Work out the finished part from the listing and answer in its coordinate system (mm). A direction names the side the tool comes from. Coordinates: 2 decimals unless noted, no trailing zeros. Write each loop counter-clockwise with the first axis right and the second up, starting at its lowest first coordinate (ties: lowest second). Pieces come first, ordered by that corner, then holes. Notation, with made-up numbers: (65.5, 52.25) - (106.5, 52.25) arc R37 ccw to (106.5, 89.25) - close; hole circle Ø1 at (-0.75, 13). An arc over 180 degrees is marked (long way). One line per item, written item: value.
```python
from build123d import *

# Parameters (mm, degrees)
F1_DEPTH = 3.41884
F2_R     = 0.762
F3_R     = 1.35255
F4_DEPTH = 3.41884


with BuildPart() as f1:
    # F0 (on Top) → F1 (new body)
    with BuildSketch(Plane.XY):
        with BuildLine():
            ThreePointArc((6.35, 0), (3.175, 3.175), (0, 0))
            Line((0, 0), (0, -169.139565))
            Line((0, -169.139565), (-3.174995, -174.638818))
            Line((-3.174995, -174.638818), (9.524995, -174.638818))
            Line((9.524995, -174.638818), (6.35, -169.139565))
            Line((6.35, -169.139565), (6.35, 0))
        make_face()
    extrude(amount=F1_DEPTH)

    # F2
    f2_edges = [f1.edges().sort_by_distance(p)[0] for p in [
        (9.524995, -174.638818, 1.70942),
        (-3.174995, -174.638818, 1.70942),
    ]]
    fillet(f2_edges, radius=F2_R)

    # F3 (on face) → F4 (cut, through all)
    with BuildSketch(Plane.XY.offset(3.41884)):
        with Locations((3.175, 0)):
            Circle(F3_R)
        with Locations((3.175, -85.731909)):
            Circle(F3_R)
        with Locations((3.175, -171.463818)):
            Circle(F3_R)
    extrude(amount=-F4_DEPTH, mode=Mode.SUBTRACT)


solid = f1.part
```
Item 1: Section B-B, the plane y = -155 is taken. Determine the outline of the cut face in (x, z), then the cut area to 3 significant figures.
Evaluation:
outline: (0, 0) - (6.35, 0) - (6.35, 3.42) - (0, 3.42) - close
area: 21.7 mm2
Item 2: Section A-A, the plane z = 1.3 is taken. Determine the outline of the cut face in (x, y) (3 decimals), then the cut area to 3 significant figures.
Evaluation:
outline: (-2.515, -173.496) arc R0.762 ccw to (-1.855, -174.639) - (8.205, -174.639) arc R0.762 ccw to (8.865, -173.496) - (6.35, -169.14) - (6.35, 0) arc R3.175 ccw to (0, 0) - (0, -169.14) - close; hole circle Ø2.705 at (3.175, -171.464); hole circle Ø2.705 at (3.175, -85.732); hole circle Ø2.705 at (3.175, 0)
area: 1,120 mm2
Item 3: Given pin 1 (1.5 mm diameter, centred on x = -1.5, z = 1.5, fed in from +Y), flat-ended and moving along its own axis, determine where the tip first touches the part or whether it passes through.
Evaluation:
pin 1: stops at y = -170.44
Item 4: Consider probe 1 along Y at (x, z) = (3.75, 0.3); probe 2 along X at (y, z) = (-11, 1); probe 3 along Y at (x, z) = (5.75, 3.1). Determine where each line is inside the solid, lowest interval first.
Evaluation:
probe 1: y = -174.64 to -172.69, -170.24 to -86.96, -84.51 to -1.22, 1.22 to 3.12
probe 2: x = 0 to 6.35
probe 3: y = -174.64 to 1.86
Item 5: Determine the mould class of faces 1 (the face through (3, -84.39, 1.73)), 2 (the face through (3, -174.639, 2)), 3 (the face through (3.245, 3.174, 1.685)), 4 (the face through (2.1, -0.82, 1.73)) for opening direction X: +X half, -X half, draft (parallel to the pull), parting line (faces both ways), or undercut.
Evaluation:
face 1: undercut
face 2: draft
face 3: parting line
face 4: undercut
Item 6: Which of the six approach directions +Z, -Z, +X, -X, +Y, -Y give full straight-line access (tool end or side, diameter ignored) to faces 5 (the face through (6.35, -86, 2)), 6 (the face through (0, -83, 2)), 7 (the face through (2, -84, 0))?
Evaluation:
face 5: +Z, -Z, +X, +Y
face 6: +Z, -Z, -X, +Y
face 7: -Z, +X, -X, +Y, -Y
